Source: CAD feature listing. Evaluate the final solid. Frame: model axes, mm. A direction names the side the tool comes from. Round coordinates to 2 decimals unless told otherwise and drop trailing zeros. Order: outer loops, then holes, each group sorted by start corner. A loop starts at its lowest first (then second) coordinate and runs counter-clockwise, first axis right, second up. Notation, with made-up numbers: (-1.5, 72.25) - (28.5, 72.25) arc R32 ccw to (28.5, 104.25) - close; hole circle Ø4 at (-32.5, 83). An arc over 180 degrees is marked (long way). Use one line per item in the form item = value. Start each with the question number.
Q1. Pin query (flat end, axial travel): pin 1 Ø3 at (x, y) = (10, 10) entering from -Z; pin 2 Ø0.5 at (y, z) = (-1, 0.5) entering from -X; pin 3 Ø0.5 at (x, z) = (-7.5, 0.5) entering from -Y. Return the tip coordinate at first contact, or that it passes through.
Q2. Ray query, line 1 (X direction, y = 10, z = 0.3); line 2 (Y direction, x = 0, z = 0.75); line 3 (X direction, y = -18.5, z = 0.95). Return the intervals inside material, ascending. Write a range as [from, to].
Q3. Cut plane A-A, the plane x = 0. Return the cut outline in (y, z), and give its area (3 significant figures).
Q4. Draft query along X for faces 1 (the cylindrical face through (0, 18, 0.5)), 2 (the flat face through (-6.1, -20, 0.5)), 3 (the cylindrical face through (10.13, 9.01, 0.51)), 4 (the flat face through (10, 15.9, 0.5)). Return one class per face: released by +X, released by -X, zero draft, split by the parting line, or undercut.
Q5. Cut plane D-D, the plane x = -6.25. Return the cut outline in (y, z), and give its area (3 significant figures).
Q6. Cut plane B-B, the plane z = 0.15. Return the cut outline in (x, y).
Q7. Set-up query: faces 5 (the flat face through (5.9, -20, 0.5)), 6 (the flat face through (-10, 0.1, 0.5)), 7 (the flat face through (-10, 16.1, 0.5)). Return all of +Z, -Z, +X, -X, +Y, -Y with unobstructed straight access to the full face (end or side cutting, diameter ignored); none if empty.
Q8. Cut plane C-C, the plane y = 10. Return the cut outline in (x, z), and give its area (3 significant figures).
from build123d import *

# Parameters (mm, degrees)
F1_DEPTH = 1
F2_D     = 4
F3_D     = 2


with BuildPart() as f1:
    # F0 (on Top) → F1 (new body)
    with BuildSketch(Plane.XY):
        with BuildLine():
            Line((10, 12), (10, 20))
            Line((10, 20), (2, 20))
            ThreePointArc((2, 20), (0, 18), (-2, 20))
            Line((-2, 20), (-10, 20))
            Line((-10, 20), (-10, 12))
            Line((-10, 12), (-10, 8))
            Line((-10, 8), (-10, -8))
            ThreePointArc((-10, -8), (-8.5857864376, -8.5857864376), (-8, -10))
            ThreePointArc((-8, -10), (-8.5857864376, -11.4142135624), (-10, -12))
            Line((-10, -12), (-10, -20))
            Line((-10, -20), (-2, -20))
            Line((-2, -20), (2, -20))
            Line((2, -20), (10, -20))
            Line((10, -20), (10, -12))
            ThreePointArc((10, -12), (8, -10), (10, -8))
            Line((10, -8), (10, 8))
            Line((10, 8), (10, 12))
        make_face()
        with BuildLine():
            ThreePointArc((-2, 20), (0, 18), (2, 20))
            Line((2, 20), (-2, 20))
        make_face()
        with BuildLine():
            Line((-2, 20), (2, 20))
            ThreePointArc((2, 20), (0, 22), (-2, 20))
        make_face()
        with BuildLine():
            ThreePointArc((10, 8), (12, 10), (10, 12))
            Line((10, 12), (10, 8))
        make_face()
        with BuildLine():
            ThreePointArc((12, -10), (11.4142135624, -8.5857864376), (10, -8))
            Line((10, -8), (10, -12))
            ThreePointArc((10, -12), (11.4142135624, -11.4142135624), (12, -10))
        make_face()
        with BuildLine():
            Line((10, -12), (10, -8))
            ThreePointArc((10, -8), (8, -10), (10, -12))
        make_face()
        with BuildLine():
            Line((-10, 8), (-10, 12))
            ThreePointArc((-10, 12), (-12, 10), (-10, 8))
        make_face()
        with BuildLine():
            ThreePointArc((-8, -10), (-8.5857864376, -8.5857864376), (-10, -8))
            Line((-10, -8), (-10, -12))
            ThreePointArc((-10, -12), (-8.5857864376, -11.4142135624), (-8, -10))
        make_face()
        with BuildLine():
            Line((-10, -12), (-10, -8))
            ThreePointArc((-10, -8), (-12, -10), (-10, -12))
        make_face()
        with BuildLine():
            ThreePointArc((-2, -20), (0, -22), (2, -20))
            Line((2, -20), (-2, -20))
        make_face()
    extrude(amount=F1_DEPTH)

    # F2 (through all)
    with Locations(Plane(origin=(0, 0, 0), x_dir=(1, 0, 0), z_dir=(0, 0, -1))):
        with Locations((0, -20), (-10, 10), (10, 10)):
            Hole(F2_D / 2)

    # F3 (through all)
    with Locations(Plane(origin=(0, 0, 0), x_dir=(1, 0, 0), z_dir=(0, 0, -1))):
        with Locations((-10, -10), (10, -10), (0, 20)):
            Hole(F3_D / 2)


solid = f1.part
Completed:
q1.pin_1 = 0
q1.pin_2 = -10
q1.pin_3 = -20
q2.line_1 = [-12, -11], [-9, 9], [11, 12]
q2.line_2 = [-22, -21], [-19, 18]
q2.line_3 = [-10, 10]
q3.outline = (-22, 0) - (-21, 0) - (-21, 1) - (-22, 1) - close; (-19, 0) - (18, 0) - (18, 1) - (-19, 1) - close
q3.area = 38.0 mm2
q4.face_1 = undercut
q4.face_2 = zero draft
q4.face_3 = undercut
q4.face_4 = released by +X
q5.outline = (-20, 0) - (20, 0) - (20, 1) - (-20, 1) - close
q5.area = 40.0 mm2
q6.outline = (-10, -20) - (-2, -20) arc R2 ccw to (2, -20) - (10, -20) - (10, -12) arc R2 cw to (10, -8) - (10, 8) arc R2 ccw to (10, 12) - (10, 20) - (2, 20) arc R2 cw to (-2, 20) - (-10, 20) - (-10, 12) arc R2 ccw to (-10, 8) - (-10, -8) arc R2 cw to (-10, -12) - close; hole circle Ø2 at (-10, 10); hole circle Ø2 at (0, -20); hole circle Ø2 at (10, 10)
q7.face_5 = +Z, -Z, +X, -Y
q7.face_6 = +Z, -Z, -X, -Y
q7.face_7 = +Z, -Z, -X, +Y
q8.outline = (-12, 0) - (-11, 0) - (-11, 1) - (-12, 1) - close; (-9, 0) - (9, 0) - (9, 1) - (-9, 1) - close; (11, 0) - (12, 0) - (12, 1) - (11, 1) - close
q8.area = 20.0 mm2
